Input: part model. Units: mm. Frame: model coordinates. Face numbers are marked on the shaded views. A direction names the side the tool comes from. Give positions to 0.01 mm unless a question says otherwise; leave off trailing zeros. Write each loop counter-clockwise with the first axis right and the second up, starting at its lowest first coordinate (ties: lowest second). Pieces come first, ordered by that corner, then holes. Notation, with made-up numbers: (74.5, 68) - (118.5, 68) arc R23 cw to (118.5, 85) - close; hole circle Ø1 at (-31, -30.5). An arc over 180 degrees is marked (long way). Answer as CSV lines item,"result". Start each with the question number.
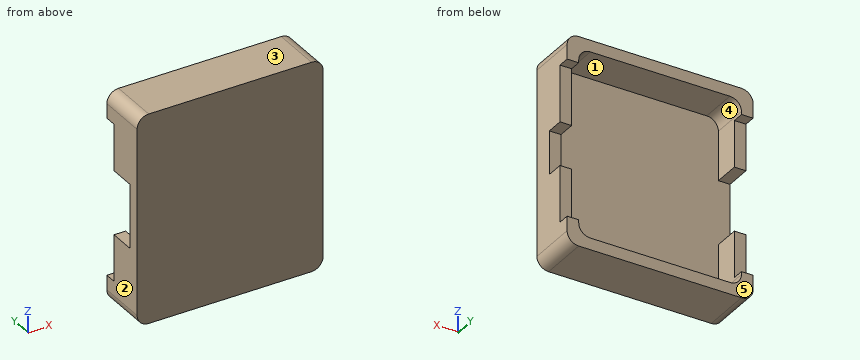
from build123d import *

# Parameters (mm, degrees)
SKETCH1_W           = 32
SKETCH1_H           = 36
BOSS_EXTRUDE1_DEPTH = 2
SKETCH2_W           = 32
SKETCH2_H           = 36
SKETCH2_W_2         = 28
SKETCH2_H_2         = 32
BOSS_EXTRUDE2_DEPTH = 6.5
CUT_EXTRUDE1_DEPTH  = 2
CUT_EXTRUDE2_DEPTH  = 2
FILLET1_R           = 2


with BuildPart() as part:
    # Sketch1 → Boss-Extrude1 (new body)
    with BuildSketch(Plane(origin=(0, 0, 0), x_dir=(1, 0, 0), z_dir=(0, 1, 0))):
        Rectangle(SKETCH1_W, SKETCH1_H)
    extrude(amount=BOSS_EXTRUDE1_DEPTH)

    # Sketch2 → Boss-Extrude2 (add)
    with BuildSketch(Plane(origin=(0, 2, 0), x_dir=(1, 0, 0), z_dir=(0, 1, 0))):
        Rectangle(SKETCH2_W, SKETCH2_H)
        Rectangle(SKETCH2_W_2, SKETCH2_H_2, mode=Mode.SUBTRACT)
    extrude(amount=BOSS_EXTRUDE2_DEPTH)

    # Sketch3 → Cut-Extrude1 (cut)
    with BuildSketch(Plane.ZY.offset(16)):
        Polygon((-13.5, 8.5), (-13.5, 6.5), (-5.5, 6.5), (-5.5, 2), (5.5, 2), (5.5, 6.5), (13.5, 6.5), (13.5, 8.5), align=None)
    extrude(amount=-CUT_EXTRUDE1_DEPTH, mode=Mode.SUBTRACT)

    # Sketch4 → Cut-Extrude2 (cut)
    with BuildSketch(Plane(origin=(16, 0, 0), x_dir=(0, 0, -1), z_dir=(1, 0, 0))):
        Polygon((-13.5, 8.5), (-13.5, 6.5), (-3.75, 6.5), (-3.75, 3.5), (3.75, 3.5), (3.75, 6.5), (13.5, 6.5), (13.5, 8.5), align=None)
    extrude(amount=-CUT_EXTRUDE2_DEPTH, mode=Mode.SUBTRACT)

    # Fillet1
    fillet1_edges = [part.edges().sort_by_distance(p)[0] for p in [
        (14, 5.25, -16),
        (14, 5.25, 16),
        (-14, 5.25, 16),
        (-14, 5.25, -16),
        (16, 4.25, 18),
        (-16, 4.25, 18),
        (-16, 4.25, -18),
        (16, 4.25, -18),
    ]]
    fillet(fillet1_edges, radius=FILLET1_R)


solid = part.part
1) Cut plane C-C on y = 5. Output: boundary loops of the cut face in (x, z).
2) Contact query for flat-ended pins moving along their axis: P1, Ø0.6, axis at x = -14.5, y = 3.5, coming from the -Z side; P2, Ø2, axis at x = 15, z = -1.5, coming from the +Y side; P3, Ø2, axis at x = 15.5, z = 10, coming from the +Y side; P4, Ø2, axis at x = -6, z = -11.5, coming from the -Y side. Output: stop coordinate, or through.
3) Cut plane B-B on z = -9. Output: boundary loops of the cut face in (x, y), and give its area (3 significant figures).
4) Cut plane D-D on x = 6. Output: boundary loops of the cut face in (y, z), and give its area (3 significant figures).
5) Material intervals for line 1 (Z direction, x = 7, y = 7.75); line 2 (X direction, y = 4.5, z = -7); line 3 (Y direction, x = 9.5, z = 13), sorted ascending. Write a range as from..to.
6) Reachability of the marked faces 4 and 5 from +Z, -Z, +X, -X, +Y, -Y: full face, straight path, thin tool, end or side. Return the list, or none.
7) Cut plane A-A on y = 7. Output: boundary loops of the cut face in (x, z).
8) Pull-direction query (Z, two-part tool) for the marked faces 1, 2 and 3; classes: +Z half, -Z half, draft (parallel to the pull), parting line (faces both ways), or undercut.
Numbers:
1,outline,"(-16, -16) arc R2 ccw to (-14, -18) - (14, -18) arc R2 ccw to (16, -16) - (16, -3.75) - (14, -3.75) - (14, -14) arc R2 cw to (12, -16) - (-12, -16) arc R2 cw to (-14, -14) - (-14, -5.5) - (-16, -5.5) - close; (-16, 5.5) - (-14, 5.5) - (-14, 14) arc R2 cw to (-12, 16) - (12, 16) arc R2 cw to (14, 14) - (14, 3.75) - (16, 3.75) - (16, 16) arc R2 ccw to (14, 18) - (-14, 18) arc R2 ccw to (-16, 16) - close"
2,P1,"stops at z = -17.99"
2,P2,"stops at y = 3.5"
2,P3,"stops at y = 6.5"
2,P4,"stops at y = 0"
3,outline,"(-16, 0) - (16, 0) - (16, 6.5) - (14, 6.5) - (14, 2) - (-14, 2) - (-14, 6.5) - (-16, 6.5) - close"
3,area,"82.0 mm²"
4,outline,"(0, -18) - (8.5, -18) - (8.5, -16) - (2, -16) - (2, 16) - (8.5, 16) - (8.5, 18) - (0, 18) - close"
4,area,"98.0 mm²"
5,line 1,"z = -18..-16, 16..18"
5,line 2,"x = -16..-14, 14..16"
5,line 3,"y = 0..2"
6,face 4,"+Y"
6,face 5,"+Z, -Z, +X, -X, +Y"
7,outline,"(-16, -16) arc R2 ccw to (-14, -18) - (14, -18) arc R2 ccw to (16, -16) - (16, -13.5) - (14, -13.5) - (14, -14) arc R2 cw to (12, -16) - (-12, -16) arc R2 cw to (-14, -14) - (-14, -13.5) - (-16, -13.5) - close; (-16, 13.5) - (-14, 13.5) - (-14, 14) arc R2 cw to (-12, 16) - (12, 16) arc R2 cw to (14, 14) - (14, 13.5) - (16, 13.5) - (16, 16) arc R2 ccw to (14, 18) - (-14, 18) arc R2 ccw to (-16, 16) - close"
8,face 1,"undercut"
8,face 2,"draft"
8,face 3,"+Z half"
